Design review of the part shown in the three views and the two pictorial views. Dimensions are in mm from the part's minimum x, y and z. Give positions to 0.01 mm unless a question says otherwise; leave off trailing zeros. Order: outer loops, then holes, each group sorted by start corner. A loop starts at its lowest first (then second) coordinate and runs counter-clockwise, first axis right, second up.
Item 1: Consider section D-D (z = 257). Give the boundary of the cut face in (x, y).
Item 2: Consider section A-A (z = 145). Give the boundary of the cut face in (x, y).
Item 3: For probe 1 along Y at (x, z) = (1.9, 230); probe 2 along Z at (x, y) = (1.55, 41); probe 3 along Z at (x, y) = (2.7, 8), list the stretches that pass through material, from the lowest coordinate up.
Item 4: For P1, Ø5, axis at y = 10.5, z = 252, coming from the -X side; P2, Ø0.9, axis at x = 1.5, z = 280.5, coming from the +Y side, all flat-tipped, find the tip position at first contact; note any pin that passes through.
Item 5: Consider section B-B (x = 2.3). Give the number of separate pieces and of enclosed holes in the cut face, plus the area to 3 significant figures.
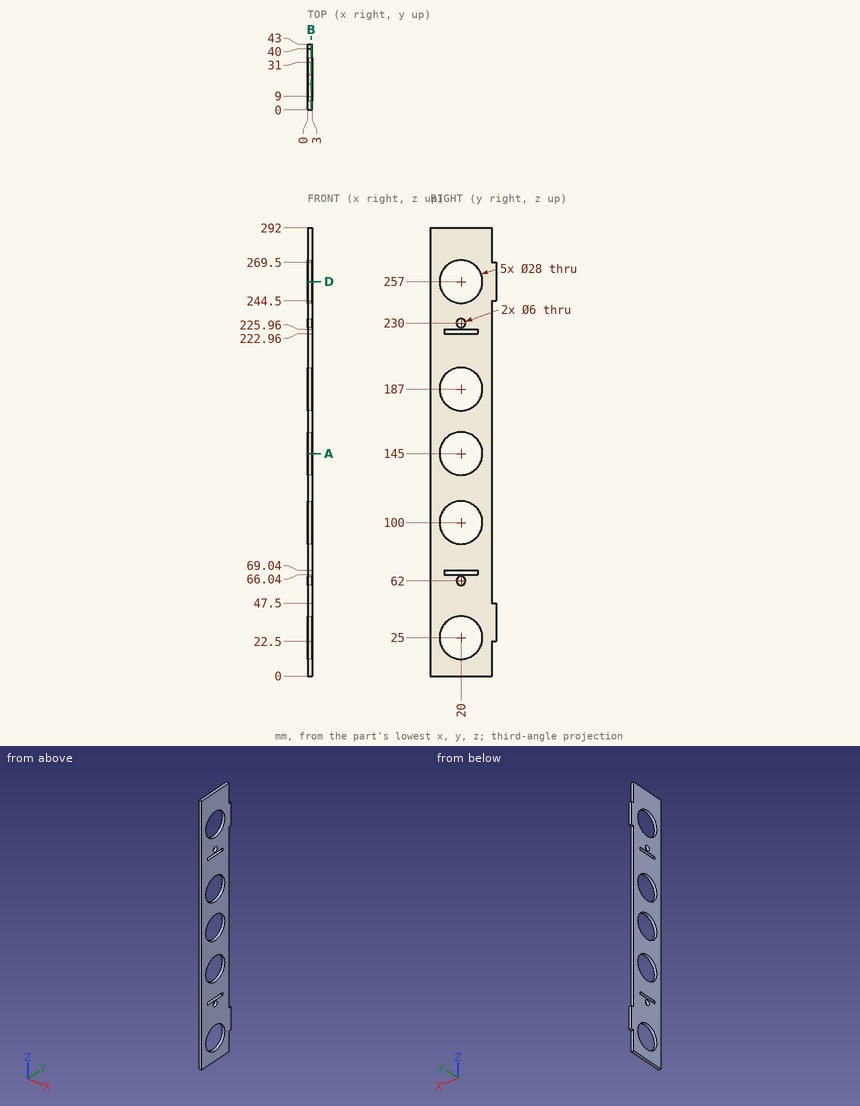
Resolved:
1. outline: (0, 0) - (3, 0) - (3, 6) - (0, 6) - close; (0, 34) - (3, 34) - (3, 43) - (0, 43) - close
2. outline: (0, 0) - (3, 0) - (3, 6) - (0, 6) - close; (0, 34) - (3, 34) - (3, 40) - (0, 40) - close
3. probe 1: y = 0 to 17, 23 to 40
3. probe 2: z = 22.5 to 47.5, 244.5 to 269.5
3. probe 3: z = 0 to 17.79, 32.21 to 92.79, 107.21 to 137.79, 152.21 to 179.79, 194.21 to 249.79, 264.21 to 292
4. P1: passes through
4. P2: stops at y = 40
5. separate pieces: 1
5. enclosed holes: 9
5. area: 8,560 mm2
